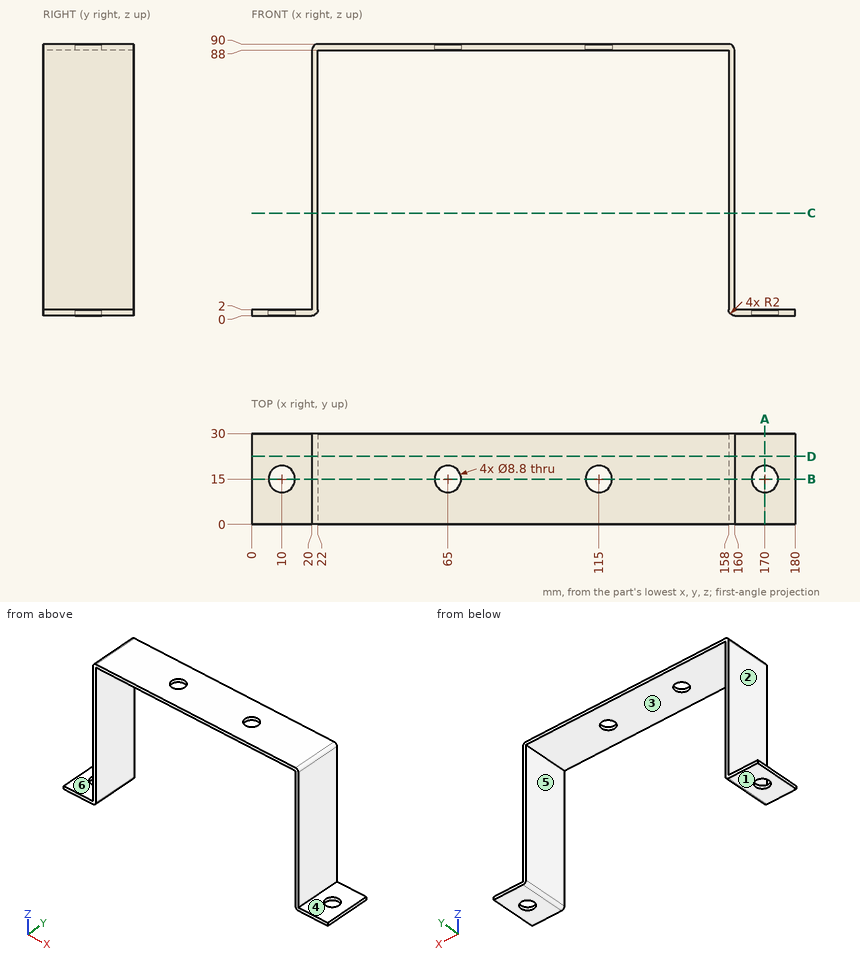
Geometry check sheet. Reference: drawing and pictorial views, mm from the part's lowest x, y, z. A direction names the side the tool comes from. Give positions to 0.01 mm unless a question says otherwise; leave off trailing zeros. Order: outer loops, then holes, each group sorted by start corner. A loop starts at its lowest first (then second) coordinate and runs counter-clockwise, first axis right, second up. Notation, with made-up numbers: M 11.25,34 L 27.25,34 A26 cw 27.25,68 Z; hole C -36,39.25 d4. An arc over 180 degrees is marked long. Return JSON: item names as keys, results as strings. Group by question number.
1) Go/stop test with flat-tipped pins: pin 1 Ø3 at (y, z) = (13.5, 33) entering from +X; pin 2 Ø6 at (x, y) = (13.5, 15) entering from +Z; pin 3 Ø3 at (y, z) = (24.5, 36) entering from -X. Record where each tip stops, or that it passes through.
2) Scan lines: line 1 (Y direction, x = 170, z = 1.4); line 2 (X direction, y = 3.5, z = 53); line 3 (Z direction, x = 103.5, y = 16.25). Record each from-to range of solid material in increasing order.
3) Access from +Z, -Z, +X, -X, +Y, -Y to the whole of each face (thin tool, end or side, straight path). Record for the marked faces 4, 5 and 6.
4) Section check B-B on y = 15. Give the number of separate pieces and of enclosed holes in the cut face, and give its area (3 significant figures).
5) Mould release check, pull along X, two halves, no side actions. Record for the marked faces 1, 2 and 3: pulls with the +X half, pulls with the -X half, needs draft (parallel to the pull), parting line crosses it, or undercut.
6) Section check D-D on y = 22.5. Record the cut outline in (x, z).
7) Section check C-C on z = 34. Record the cut outline in (x, y), and give its area (3 significant figures).
8) Section check A-A on x = 170. Record the cut outline in (y, z).
Answer block:
{
 "1": {"pin 1": "stops at x = 160", "pin 2": "stops at z = 2", "pin 3": "stops at x = 20"},
 "2": {"line 1": "y = 0 to 10.6, 19.4 to 30", "line 2": "x = 20 to 22, 158 to 160", "line 3": "z = 88 to 90"},
 "3": {"face 4": "+Z, +X, +Y, -Y", "face 5": "-Z, +Y, -Y", "face 6": "+Z, -X, +Y, -Y"},
 "4": {"separate pieces": "5", "enclosed holes": "0", "area": "638 mm^2"},
 "5": {"face 1": "needs draft", "face 2": "pulls with the -X half", "face 3": "undercut"},
 "6": {"outline": "M 0,0 L 20,0 A2 ccw 22,2 L 22,88 L 158,88 L 158,2 A2 ccw 160,0 L 180,0 L 180,2 L 160,2 L 160,88 A2 ccw 158,90 L 22,90 A2 ccw 20,88 L 20,2 L 0,2 Z"},
 "7": {"outline": "M 20,0 L 22,0 L 22,30 L 20,30 Z; M 158,0 L 160,0 L 160,30 L 158,30 Z", "area": "120 mm^2"},
 "8": {"outline": "M 0,0 L 10.6,0 L 10.6,2 L 0,2 Z; M 19.4,0 L 30,0 L 30,2 L 19.4,2 Z"}
}
